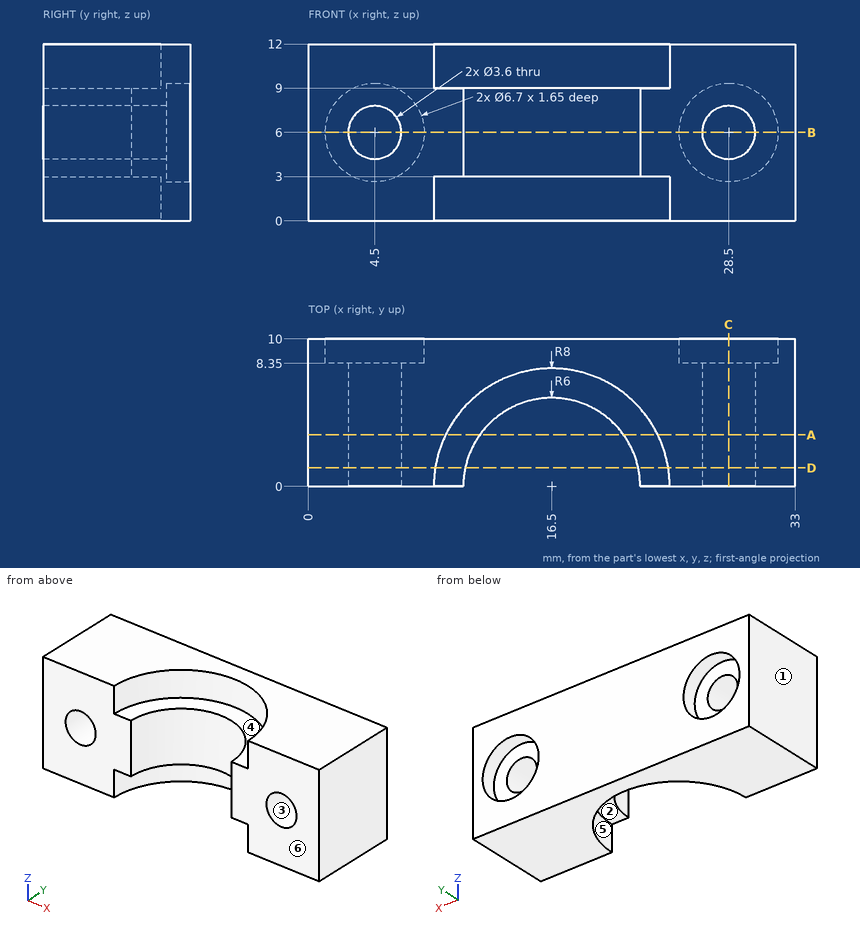
Answer from the drawing. Dimensions are ordinates in mm from the lowest x, y and z of the part. A direction names the side the tool comes from. Coordinates: 2 decimals unless noted, no trailing zeros. Loops run counter-clockwise (first coordinate to the right, second up) from the corner with the lowest first, then second, coordinate; pieces in that order, holes last. Notation, with made-up numbers: (-33.75, 57) - (3.25, 57) arc R16 cw to (3.25, 86) - close; hole circle Ø11 at (51.25, 24). An arc over 180 degrees is marked (long way). Answer in a Markdown table with one row per item.
1. Find section D-D, the plane y = 1.25. Write down the section's boundary in (x, z), then the cut area to 3 significant figures.
Conclusion:
| item | result |
|---|---|
| outline | (0, 0) - (8.6, 0) - (8.6, 3) - (10.63, 3) - (10.63, 9) - (8.6, 9) - (8.6, 12) - (0, 12) - close; (22.37, 3) - (24.4, 3) - (24.4, 0) - (33, 0) - (33, 12) - (24.4, 12) - (24.4, 9) - (22.37, 9) - close; hole circle Ø3.6 at (4.5, 6); hole circle Ø3.6 at (28.5, 6) |
| area | 210 mm² |
2. Given pin 1 (2.5 mm diameter, centred on x = 13, y = 4, fed in from -Z); pin 2 (2 mm diameter, centred on x = 13.5, z = 6.5, fed in from -Y), each flat-ended and moving along its own axis, determine where each tip first touches the part or whether it passes through.
Conclusion:
| item | result |
|---|---|
| pin 1 | stops at z = 3 |
| pin 2 | stops at y = 4.47 |
3. Find section A-A, the plane y = 3.5. Write down the section's boundary in (x, z), then the cut area to 3 significant figures.
Conclusion:
| item | result |
|---|---|
| outline | (0, 0) - (9.31, 0) - (9.31, 3) - (11.63, 3) - (11.63, 9) - (9.31, 9) - (9.31, 12) - (0, 12) - close; (21.37, 3) - (23.69, 3) - (23.69, 0) - (33, 0) - (33, 12) - (23.69, 12) - (23.69, 9) - (21.37, 9) - close; hole circle Ø3.6 at (4.5, 6); hole circle Ø3.6 at (28.5, 6) |
| area | 231 mm² |
4. Straight lines are drawn through the part: line 1 (X direction, y = 8.7, z = 6); line 2 (X direction, y = 4.5, z = 6); line 3 (X direction, y = 4.25, z = 6). For each, find the intervals that lie inside material, in ascending order.
Conclusion:
| item | result |
|---|---|
| line 1 | x = 0 to 1.15, 7.85 to 25.15, 31.85 to 33 |
| line 2 | x = 0 to 2.7, 6.3 to 12.53, 20.47 to 26.7, 30.3 to 33 |
| line 3 | x = 0 to 2.7, 6.3 to 12.26, 20.74 to 26.7, 30.3 to 33 |
5. Find section B-B, the plane z = 6. Write down the section's boundary in (x, y), then the cut area to 3 significant figures.
Conclusion:
| item | result |
|---|---|
| outline | (0, 0) - (2.7, 0) - (2.7, 8.35) - (1.15, 8.35) - (1.15, 10) - (0, 10) - close; (6.3, 0) - (10.5, 0) arc R6 cw to (22.5, 0) - (26.7, 0) - (26.7, 8.35) - (25.15, 8.35) - (25.15, 10) - (7.85, 10) - (7.85, 8.35) - (6.3, 8.35) - close; (30.3, 0) - (33, 0) - (33, 10) - (31.85, 10) - (31.85, 8.35) - (30.3, 8.35) - close |
| area | 191 mm² |
6. Determine the mould class of the marked faces 1, 2 and 3 for opening direction Z: +Z half, -Z half, draft (parallel to the pull), parting line (faces both ways), or undercut.
Conclusion:
| item | result |
|---|---|
| face 1 | draft |
| face 2 | -Z half |
| face 3 | undercut |
7. Find section C-C, the plane x = 28.5. Write down the section's boundary in (y, z), then the cut area to 3 significant figures.
Conclusion:
| item | result |
|---|---|
| outline | (0, 0) - (10, 0) - (10, 2.65) - (8.35, 2.65) - (8.35, 4.2) - (0, 4.2) - close; (0, 7.8) - (8.35, 7.8) - (8.35, 9.35) - (10, 9.35) - (10, 12) - (0, 12) - close |
| area | 78.9 mm² |
8. Which of the six approach directions +Z, -Z, +X, -X, +Y, -Y give full straight-line access (tool end or side, diameter ignored) to the marked faces 4, 5 and 6?
Conclusion:
| item | result |
|---|---|
| face 4 | +Z, -Y |
| face 5 | -Z, -Y |
| face 6 | +Z, -Z, +X, -X, -Y |
